Can you work these out from the model? Positions are in its coordinate system, mm. Face numbers are marked on the shaded views. A direction names the side the tool comes from. Coordinates: 2 decimals unless noted, no trailing zeros. Order: outer loops, then holes, each group sorted by start corner. A loop starts at its lowest first (then second) coordinate and runs counter-clockwise, first axis right, second up. Notation, with made-up numbers: M 17.25,-1 L 38.25,-1 A24 cw 38.25,16 Z; hole C -28,-8.5 d8. An arc over 180 degrees is marked long. Answer as a JSON object with one key per item and string values.
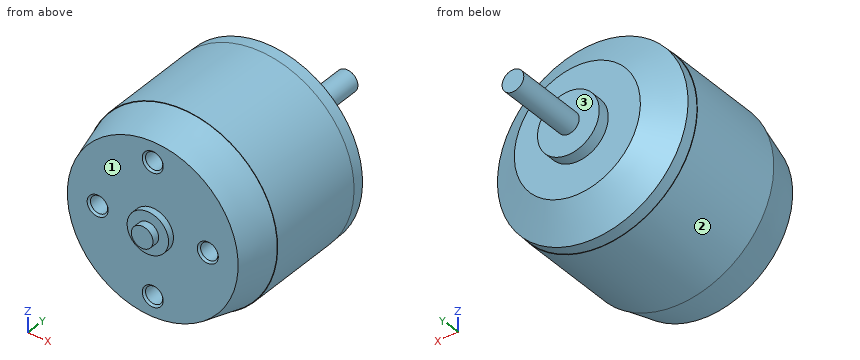
from build123d import *

# Parameters (mm, degrees)
M3X0_5_TAPPED_HOLE1_D           = 2.5
M3X0_5_TAPPED_HOLE1_DEPTH       = 7.499985
M3X0_5_TAPPED_HOLE1_CSINK_D     = 3.05
M3X0_5_TAPPED_HOLE1_CSINK_ANGLE = 90
M3X0_5_TAPPED_HOLE1_TIP         = 0.751075774
M3X0_5_TAPPED_HOLE2_D           = 2.5
M3X0_5_TAPPED_HOLE2_DEPTH       = 7.499985
M3X0_5_TAPPED_HOLE2_CSINK_D     = 3.05
M3X0_5_TAPPED_HOLE2_CSINK_ANGLE = 90
M3X0_5_TAPPED_HOLE2_TIP         = 0.751075774
SKETCH11_W                      = 13.9065
SKETCH11_H                      = 14.8717


with BuildPart() as part:
    # Sketch4 → Revolve1 (revolve)
    with BuildSketch(Plane.XY, mode=Mode.PRIVATE) as revolve1_sk:
        Polygon((0, 0), (1.5748, 0), (1.5748, 1.1049), (3.0099, 1.1049), (3.0099, 2.0574), (12.4079, 2.0574), (13.843, 7.747), (13.843, 24.3586), (9.1567, 27.3558), (4.4831, 27.3558), (4.4831, 29.1084), (1.5748, 29.1084), (1.5748, 39.9034), (0, 39.9034), align=None)
    revolve(revolve1_sk.sketch.rotate(Axis((0, -72.371810048, 0), (0, 1, 0)), 90), axis=Axis((0, -72.371810048, 0), (0, 1, 0)))

    # M3x0.5 Tapped Hole1
    with Locations(Plane(origin=(0, 2.0574, 0), x_dir=(-1, 0, 0), z_dir=(0, -1, 0))):
        with Locations((8, 0), (-8, 0)):
            CounterSinkHole(M3X0_5_TAPPED_HOLE1_D / 2, M3X0_5_TAPPED_HOLE1_CSINK_D / 2, depth=M3X0_5_TAPPED_HOLE1_DEPTH, counter_sink_angle=M3X0_5_TAPPED_HOLE1_CSINK_ANGLE)
            with Locations((0, 0, -(M3X0_5_TAPPED_HOLE1_DEPTH + M3X0_5_TAPPED_HOLE1_TIP / 2))):  # 118° drill point
                Cone(0, M3X0_5_TAPPED_HOLE1_D / 2, M3X0_5_TAPPED_HOLE1_TIP, mode=Mode.SUBTRACT)

    # M3x0.5 Tapped Hole2
    with Locations(Plane(origin=(0, 2.0574, 0), x_dir=(-1, 0, 0), z_dir=(0, -1, 0))):
        with Locations((0, 9.5), (0, -9.5)):
            CounterSinkHole(M3X0_5_TAPPED_HOLE2_D / 2, M3X0_5_TAPPED_HOLE2_CSINK_D / 2, depth=M3X0_5_TAPPED_HOLE2_DEPTH, counter_sink_angle=M3X0_5_TAPPED_HOLE2_CSINK_ANGLE)
            with Locations((0, 0, -(M3X0_5_TAPPED_HOLE2_DEPTH + M3X0_5_TAPPED_HOLE2_TIP / 2))):  # 118° drill point
                Cone(0, M3X0_5_TAPPED_HOLE2_D / 2, M3X0_5_TAPPED_HOLE2_TIP, mode=Mode.SUBTRACT)

    # Sketch11 → Revolve2 (revolve)
    with BuildSketch(Plane.XY, mode=Mode.PRIVATE) as revolve2_sk:
        with Locations((6.95325, 15.18285)):
            Rectangle(SKETCH11_W, SKETCH11_H)
    revolve(revolve2_sk.sketch.rotate(Axis((0, -72.371810048, 0), (0, 1, 0)), 90), axis=Axis((0, -72.371810048, 0), (0, 1, 0)))


solid = part.part
Item 1: Which directions (+Z, -Z, +X, -X, +Y, -Y) give clear straight access to the entire face, cutting with the end or side of a thin tool? Please do the marked faces 1, 2 and 3.
Answers follow:
{"face 1": "-Y", "face 2": "+Y, -Y", "face 3": "+Y"}
Item 2: I want a section at A-A, the plane y = 15. Write out the boundary of the cut face in (x, z).
Answers follow:
{"outline": "C 0,0 d27.81"}
Item 3: I'm going to push flat-ended pins straight in: pin 1 (8 mm diameter, centred on y = 27, z = 6, fed in from +X); pin 2 (0.8 mm diameter, centred on x = 0, z = -9, fed in from -Y); pin 3 (3 mm diameter, centred on x = 0, z = 9.5, fed in from +Y); pin 4 (9 mm diameter, centred on x = -3.5, z = 3, fed in from +Y). Where does each tip first touch, or does it pass through?
Answers follow:
{"pin 1": "stops at x = 13.51", "pin 2": "stops at y = 7.75", "pin 3": "stops at y = 27.36", "pin 4": "stops at y = 39.9"}
Item 4: Please list where these lines run through material, in increasing order: line 1 (Y direction, x = 6.5, z = 0.5); line 2 (X direction, y = 6.5, z = 9.5); line 3 (Z direction, x = -8, y = 4.4).
Answers follow:
{"line 1": "y = 2.06 to 27.36", "line 2": "x = -9.63 to -1.25, 1.25 to 9.63", "line 3": "z = -10.25 to -1.25, 1.25 to 10.25"}
